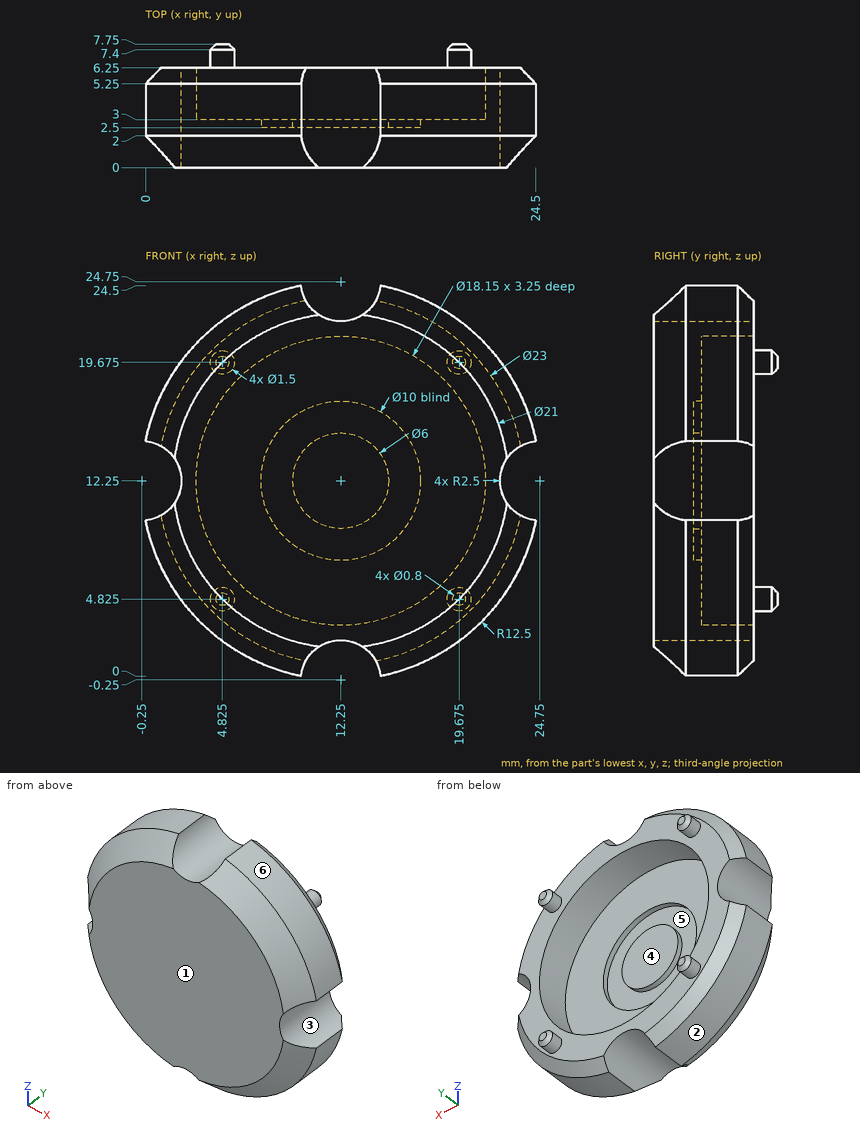
Verification items for this drawing (mm, ordinates from the low corner). A direction names the side the tool comes from. Coordinates: 2 decimals unless noted, no trailing zeros. Use one line per item in the form item = value. Start each with the question number.
Item 1: Tool access check on the marked faces 5 and 6. Record the directions out of +Z, -Z, +X, -X, +Y, -Y that give a thin tool (end or side, any length) a straight path to the whole face; none if there is none.
Item 2: Mould release check, pull along Z, two halves, no side actions. Record for the marked faces 1, 2, 3 and 4: +Z half, -Z half, draft (parallel to the pull), parting line (faces both ways), or undercut.
Item 3: Gauge pin test, flat end, axial feed: pin 1 (6.5 mm diameter, centred on x = 13, z = 11, fed in from +Y). Record the tip position at first contact, or that the pin passes through.
Item 4: Thickness scan on probe 1 along Z at (x, y) = (12.25, 2.9); probe 2 along Z at (x, y) = (19.75, 7.25); probe 3 along Y at (x, z) = (16.5, 10). Record the ranges inside material, lowest first.
Computed:
q1.face_5 = +Y
q1.face_6 = +Z, +X, +Y, -Y
q2.face_1 = draft
q2.face_2 = -Z half
q2.face_3 = undercut
q2.face_4 = undercut
q3.pin_1 = 3
q4.probe_1 = 2.25 to 7.25, 9.25 to 15.25, 17.25 to 22.25
q4.probe_2 = 4.08 to 5.57, 18.93 to 20.42
q4.probe_3 = 0 to 2.5
